For this review, take the finished solid that the model builds, in its own axes (mm). A direction names the side the tool comes from. Give positions to 0.01 mm unless a question says otherwise; leave off trailing zeros. Order: outer loops, then holes, each group sorted by start corner. A loop starts at its lowest first (then second) coordinate and runs counter-clockwise, first axis right, second up.
Item 1: For P1, Ø5, axis at x = 12, z = 4, coming from the -Y side, flat-tipped, find the tip position at first contact; note if it passes through.
Item 2: Consider section A-A (y = 4). Give the boundary of the cut face in (x, z), plus the area to 3 significant figures.
Item 3: For probe 1 along Z at (x, y) = (14.5, 3.25); probe 2 along Y at (x, z) = (27.25, 6.75); probe 3 along Z at (x, y) = (13.25, 13.5), list the stretches that pass through material, from the lowest coordinate up.
Item 4: Consider section B-B (x = 17). Give the boundary of the cut face in (y, z).
Item 5: Consider section C-C (z = -0.75). Give the boundary of the cut face in (x, y).
Item 6: Consider section D-D (y = 16). Give the boundary of the cut face in (x, z).
Item 7: Machinability: for faces 1 (the flat face through (17, 17, 0)), 2 (the cylindrical face through (17.4, 14.43, -9.24)), which of the approach directions +Z, -Z, +X, -X, +Y, -Y give a long, thin tool a straight path to every point of the face, cutting with its end or side? Answer none if there is none.
Item 8: The part is to be moulded in two halves that separate along Z. For faces 3 (the flat face through (17, 7, -12.84)), 4 (the flat face through (17, 0, 11)), 5 (the flat face through (17, 6, -9.84)), say which applies: released by +Z, released by -Z, zero draft, split by the parting line, or undercut.
```python
from build123d import *

# Parameters (mm, degrees)
ESQUISSE2_W             = 22.15
ESQUISSE2_H             = 25
BOSS_EXTRU_1_DEPTH      = 17
ESQUISSE3_W             = 22.15
ESQUISSE3_H             = 19
ENL_V_MAT_EXTRU_1_DEPTH = 15
CONG_1_R                = 2
CONG_2_R                = 2


with BuildPart() as part:
    # Esquisse2 → Boss.-Extru.1 (new body)
    with BuildSketch(Plane(origin=(0, 0, 0), x_dir=(1, 0, 0), z_dir=(0, 1, 0))):
        with Locations((17.241326531, 0.340136054)):
            Rectangle(ESQUISSE2_W, ESQUISSE2_H)
    extrude(amount=BOSS_EXTRU_1_DEPTH)

    # Esquisse3 → Enlèv. mat.-Extru.1 (cut)
    with BuildSketch(Plane.XZ):
        with Locations((17.241326531, -0.340136054)):
            Rectangle(ESQUISSE3_W, ESQUISSE3_H)
    extrude(amount=-ENL_V_MAT_EXTRU_1_DEPTH, mode=Mode.SUBTRACT)

    # Congé1
    cong_1_edges = [part.edges().sort_by_distance(p)[0] for p in [
        (17.241326531, 15, 9.159863946),
        (17.241326531, 15, -9.840136054),
    ]]
    fillet(cong_1_edges, radius=CONG_1_R)

    # Congé2
    cong_2_edges = [part.edges().sort_by_distance(p)[0] for p in [
        (17.241326531, 17, -12.840136054),
        (17.241326531, 17, 12.159863946),
    ]]
    fillet(cong_2_edges, radius=CONG_2_R)


solid = part.part
```
Resolved:
1. P1: stops at y = 15
2. outline: (6.17, -12.84) - (28.32, -12.84) - (28.32, -9.84) - (6.17, -9.84) - close; (6.17, 9.16) - (28.32, 9.16) - (28.32, 12.16) - (6.17, 12.16) - close
2. area: 133 mm2
3. probe 1: z = -12.84 to -9.84, 9.16 to 12.16
3. probe 2: y = 15 to 17
3. probe 3: z = -12.84 to -9.78, 9.1 to 12.16
4. outline: (0, -12.84) - (15, -12.84) arc R2 ccw to (17, -10.84) - (17, 10.16) arc R2 ccw to (15, 12.16) - (0, 12.16) - (0, 9.16) - (13, 9.16) arc R2 cw to (15, 7.16) - (15, -7.84) arc R2 cw to (13, -9.84) - (0, -9.84) - close
5. outline: (6.17, 15) - (28.32, 15) - (28.32, 17) - (6.17, 17) - close
6. outline: (6.17, -12.57) - (28.32, -12.57) - (28.32, 11.89) - (6.17, 11.89) - close
7. face 1: +Z, -Z, +X, -X, +Y
7. face 2: +X, -X, -Y
8. face 3: released by -Z
8. face 4: zero draft
8. face 5: undercut
